```python
from build123d import *

# Parameters (mm, degrees)
F0_W         = 9.525
F0_H         = 50.8
F0_R         = 3.175
F0_W_2       = 31.75
F0_H_2       = 31.75
F0_R_2       = 6.35
F0_H_3       = 38.1
F1_DEPTH     = 12.7
F2_R         = 3.175
F3_W         = 9.525
F3_H         = 12.7
F1_FACE1_R   = 6.35
F1_FACE1_R_2 = 3.175
F4_DEPTH     = 1.5875
F5_DEPTH     = 1.5875
F6_DEPTH     = 1.5875


with BuildPart() as f1:
    # F0 (on Right) → F1 (new body)
    with BuildSketch(Plane.YZ):
        with Locations((134.9375, 25.4)):
            Rectangle(F0_W, F0_H)
        with BuildLine():
            Line((139.7, 50.8), (139.7, 0))
            Line((139.7, 0), (304.8, 0))
            Line((304.8, 0), (304.8, 19.05))
            Line((304.8, 19.05), (266.7, 19.05))
            Line((266.7, 19.05), (266.7, 40.9178125))
            Line((266.7, 40.9178125), (290.922752809, 52.7264044944))
            ThreePointArc((290.922752809, 52.7264044944), (299.6985955056, 78.197752809), (274.227247191, 86.9735955056))
            Line((274.227247191, 86.9735955056), (200.025, 50.8))
            Line((200.025, 50.8), (139.7, 50.8))
        make_face()
        with Locations((230.1875, 12.7)):
            Circle(F0_R, mode=Mode.SUBTRACT)
        with Locations((165.1, 25.4)):
            Rectangle(F0_W_2, F0_H_2, mode=Mode.SUBTRACT)
        with BuildLine():
            Line((190.5, 38.1), (200.025, 38.1))
            ThreePointArc((200.025, 38.1), (203.2, 34.925), (200.025, 31.75))
            Line((200.025, 31.75), (200.025, 19.05))
            ThreePointArc((200.025, 19.05), (203.2, 15.875), (200.025, 12.7))
            Line((200.025, 12.7), (190.5, 12.7))
            ThreePointArc((190.5, 12.7), (187.325, 15.875), (190.5, 19.05))
            Line((190.5, 19.05), (190.5, 31.75))
            ThreePointArc((190.5, 31.75), (187.325, 34.925), (190.5, 38.1))
        make_face(mode=Mode.SUBTRACT)
        with Locations((282.575, 69.85)):
            Circle(F0_R_2, mode=Mode.SUBTRACT)
        with BuildLine():
            Line((73.025, 38.1), (73.025, 0))
            Line((73.025, 0), (130.175, 0))
            Line((130.175, 0), (130.175, 50.8))
            Line((130.175, 50.8), (73.025, 50.8))
            Line((73.025, 50.8), (73.025, 44.6185247588))
            ThreePointArc((73.025, 44.6185247588), (76.2842623794, 41.3592623794), (73.025, 38.1))
        make_face()
        with Locations((104.775, 25.4)):
            Rectangle(F0_W_2, F0_H_2, mode=Mode.SUBTRACT)
        with Locations((68.2625, 19.05)):
            Rectangle(F0_W, F0_H_3)
        with BuildLine():
            Line((0, 41.275), (0, 0))
            Line((0, 0), (63.5, 0))
            Line((63.5, 0), (63.5, 38.1))
            ThreePointArc((63.5, 38.1), (60.325, 41.275), (63.5, 44.45))
            Line((63.5, 44.45), (63.5, 50.8))
            Line((63.5, 50.8), (50.8, 50.8))
            Line((50.8, 50.8), (50.8, 25.4))
            ThreePointArc((50.8, 25.4), (44.45, 19.05), (38.1, 25.4))
            Line((38.1, 25.4), (38.1, 50.8))
            Line((38.1, 50.8), (26.7157145118, 50.8))
            Line((26.7157145118, 50.8), (0, 41.275))
        make_face()
    extrude(amount=F1_DEPTH)

    # F2
    f2_edges = [f1.edges().sort_by_distance(p)[0] for p in [
        (6.35, 200.025, 50.8),
        (6.35, 266.7, 40.917813),
        (6.35, 266.7, 19.05),
        (6.35, 304.8, 19.05),
        (6.35, 304.8, 0),
        (6.35, 149.225, 41.275),
        (6.35, 88.9, 41.275),
        (6.35, 180.975, 9.525),
        (6.35, 180.975, 41.275),
        (6.35, 120.65, 41.275),
        (6.35, 149.225, 9.525),
        (6.35, 88.9, 9.525),
        (6.35, 120.65, 9.525),
        (6.35, 26.715715, 50.8),
    ]]
    fillet(f2_edges, radius=F2_R)

    # F3 (on face) + F1_face1 (on face) → F4 (cut)
    with BuildSketch(Plane(origin=(0, 0, 0), x_dir=(0, -1, 0), z_dir=(-1, 0, 0))):
        with Locations((-195.2625, 6.35)):
            Rectangle(F3_W, F3_H)
        with BuildLine():
            Line((-190.5, 38.1), (-190.5, 50.8))
            Line((-190.5, 50.8), (-199.2923076923, 50.8))
            ThreePointArc((-199.2923076923, 50.8), (-199.6611512097, 50.8214972713), (-200.025, 50.8856979781))
            Line((-200.025, 50.8856979781), (-200.025, 38.1))
            Line((-200.025, 38.1), (-190.5, 38.1))
        make_face()
    with BuildSketch(Plane(origin=(12.7, 165.3857306848, 30.2558551576), x_dir=(0, 1, 0), z_dir=(1, 0, 0))):
        with BuildLine():
            Line((139.4142693152, -27.0808551576), (139.4142693152, -14.3808551576))
            ThreePointArc((139.4142693152, -14.3808551576), (138.4843333455, -12.1357911273), (136.2392693152, -11.2058551576))
            Line((136.2392693152, -11.2058551576), (104.4892693152, -11.2058551576))
            ThreePointArc((104.4892693152, -11.2058551576), (102.2442052849, -10.2759191878), (101.3142693152, -8.0308551576))
            Line((101.3142693152, -8.0308551576), (101.3142693152, 8.6775823424))
            ThreePointArc((101.3142693152, 8.6775823424), (101.7968747, 10.3603289769), (103.0979771804, 11.5315149267))
            Line((103.0979771804, 11.5315149267), (125.5370221242, 22.4705493368))
            ThreePointArc((125.5370221242, 22.4705493368), (134.3128648208, 47.9418976514), (108.8415165062, 56.717740348))
            Line((108.8415165062, 56.717740348), (35.2978691423, 20.8652122582))
            ThreePointArc((35.2978691423, 20.8652122582), (34.6205059413, 20.6254527961), (33.9065770075, 20.5441448424))
            Line((33.9065770075, 20.5441448424), (-92.3607306848, 20.5441448424))
            Line((-92.3607306848, 20.5441448424), (-92.3607306848, 14.3626696012))
            ThreePointArc((-92.3607306848, 14.3626696012), (-89.1014683054, 11.1034072218), (-92.3607306848, 7.8441448424))
            Line((-92.3607306848, 7.8441448424), (-101.8857306848, 7.8441448424))
            ThreePointArc((-101.8857306848, 7.8441448424), (-105.0607306848, 11.0191448424), (-101.8857306848, 14.1941448424))
            Line((-101.8857306848, 14.1941448424), (-101.8857306848, 20.5441448424))
            Line((-101.8857306848, 20.5441448424), (-114.5857306848, 20.5441448424))
            Line((-114.5857306848, 20.5441448424), (-114.5857306848, -4.8558551576))
            ThreePointArc((-114.5857306848, -4.8558551576), (-120.9357306848, -11.2058551576), (-127.2857306848, -4.8558551576))
            Line((-127.2857306848, -4.8558551576), (-127.2857306848, 20.5441448424))
            Line((-127.2857306848, 20.5441448424), (-138.120948876, 20.5441448424))
            ThreePointArc((-138.120948876, 20.5441448424), (-138.661985551, 20.4977075022), (-139.1871958927, 20.3597538606))
            Line((-139.1871958927, 20.3597538606), (-165.3857306848, 11.0191448424))
            Line((-165.3857306848, 11.0191448424), (-165.3857306848, -30.2558551576))
            Line((-165.3857306848, -30.2558551576), (136.2392693152, -30.2558551576))
            ThreePointArc((136.2392693152, -30.2558551576), (138.4843333455, -29.3259191878), (139.4142693152, -27.0808551576))
        make_face()
        with Locations((117.1892693152, 39.5941448424)):
            Circle(F1_FACE1_R, mode=Mode.SUBTRACT)
        with Locations((64.8017693152, -17.5558551576)):
            Circle(F1_FACE1_R_2, mode=Mode.SUBTRACT)
        with BuildLine():
            Line((34.6392693152, -17.5558551576), (25.1142693152, -17.5558551576))
            ThreePointArc((25.1142693152, -17.5558551576), (21.9392693152, -14.3808551576), (25.1142693152, -11.2058551576))
            Line((25.1142693152, -11.2058551576), (25.1142693152, 1.4941448424))
            ThreePointArc((25.1142693152, 1.4941448424), (21.9392693152, 4.6691448424), (25.1142693152, 7.8441448424))
            Line((25.1142693152, 7.8441448424), (34.6392693152, 7.8441448424))
            ThreePointArc((34.6392693152, 7.8441448424), (37.8142693152, 4.6691448424), (34.6392693152, 1.4941448424))
            Line((34.6392693152, 1.4941448424), (34.6392693152, -11.2058551576))
            ThreePointArc((34.6392693152, -11.2058551576), (37.8142693152, -14.3808551576), (34.6392693152, -17.5558551576))
        make_face(mode=Mode.SUBTRACT)
        with BuildLine():
            Line((-16.1607306848, -17.5558551576), (-16.1607306848, 7.8441448424))
            ThreePointArc((-16.1607306848, 7.8441448424), (-15.2307947151, 10.0892088727), (-12.9857306848, 11.0191448424))
            Line((-12.9857306848, 11.0191448424), (12.4142693152, 11.0191448424))
            ThreePointArc((12.4142693152, 11.0191448424), (14.6593333455, 10.0892088727), (15.5892693152, 7.8441448424))
            Line((15.5892693152, 7.8441448424), (15.5892693152, -17.5558551576))
            ThreePointArc((15.5892693152, -17.5558551576), (14.6593333455, -19.8009191878), (12.4142693152, -20.7308551576))
            Line((12.4142693152, -20.7308551576), (-12.9857306848, -20.7308551576))
            ThreePointArc((-12.9857306848, -20.7308551576), (-15.2307947151, -19.8009191878), (-16.1607306848, -17.5558551576))
        make_face(mode=Mode.SUBTRACT)
        with BuildLine():
            Line((-47.9107306848, -20.7308551576), (-73.3107306848, -20.7308551576))
            ThreePointArc((-73.3107306848, -20.7308551576), (-75.5557947151, -19.8009191878), (-76.4857306848, -17.5558551576))
            Line((-76.4857306848, -17.5558551576), (-76.4857306848, 7.8441448424))
            ThreePointArc((-76.4857306848, 7.8441448424), (-75.5557947151, 10.0892088727), (-73.3107306848, 11.0191448424))
            Line((-73.3107306848, 11.0191448424), (-47.9107306848, 11.0191448424))
            ThreePointArc((-47.9107306848, 11.0191448424), (-45.6656666545, 10.0892088727), (-44.7357306848, 7.8441448424))
            Line((-44.7357306848, 7.8441448424), (-44.7357306848, -17.5558551576))
            ThreePointArc((-44.7357306848, -17.5558551576), (-45.6656666545, -19.8009191878), (-47.9107306848, -20.7308551576))
        make_face(mode=Mode.SUBTRACT)
    extrude(amount=-F4_DEPTH, dir=(-1, 0, 0), mode=Mode.SUBTRACT)

    # F0 (on Right) → F5 (cut)
    with BuildSketch(Plane.YZ):
        with Locations((134.9375, 25.4)):
            Rectangle(F0_W, F0_H)
    extrude(amount=F5_DEPTH, mode=Mode.SUBTRACT)

    # F0 (on Right) → F6 (cut)
    with BuildSketch(Plane.YZ):
        with Locations((68.2625, 19.05)):
            Rectangle(F0_W, F0_H_3)
    extrude(amount=F6_DEPTH, mode=Mode.SUBTRACT)


solid = f1.part
```
Here's how the part is built. I have some questions about the finished solid (model axes, mm). A direction names the side the tool comes from. Coordinates: 2 decimals unless noted, no trailing zeros. Order: outer loops, then holes, each group sorted by start corner. A loop starts at its lowest first (then second) coordinate and runs counter-clockwise, first axis right, second up.
1) We'd pull the mould along Z, two halves only. Please class faces 4 (the face through (6, 33, 50.8)), 5 (the face through (1.588, 68, 19)), 6 (the face through (6, 88.9, 25)): +Z half, -Z half, draft (parallel to the pull), parting line (faces both ways), or undercut.
2) Imagine slicing it at C-C on y = 249. List the corners of the cut face in (x, z) for me.
3) Imagine slicing it at A-A on z = 69.85. List the corners of the cut face in (x, y) for me (3 decimals), and give its area (3 significant figures).
4) Will these pins go through, and if not, where does the flat tip stop? pin 1 (7.5 mm diameter, centred on y = 282.575, z = 69.85, fed in from -X) (1 decimal); pin 2 (5 mm diameter, centred on x = 5.5, y = 196, fed in from +Z); pin 3 (4 mm diameter, centred on x = 9, y = 279.5, fed in from +Z); pin 4 (2 mm diameter, centred on x = 7, z = 78, fed in from +Y).
5) Which directions (+Z, -Z, +X, -X, +Y, -Y) give clear straight access to the entire face, cutting with the end or side of a thin tool? Please do faces 1 (the face through (6, 57, 50.8)), 2 (the face through (6, 165, 9.525)), 3 (the face through (1.588, 195, 45)).
6) I need wall thicknesses on line 1 (Y direction, x = 9.5, z = 30) (3 decimals); line 2 (Z direction, x = 9.25, y = 108) (3 decimals); line 3 (Z direction, x = 10, y = 194). Which ranges of each line are inside material? Lowest first, please.
7) Imagine slicing it at B-B on x = 5. State how many separate pieces and enclosed holes the cut face has, and give its area (3 significant figures).
8) Imagine slicing it at D-D on y = 18. List the corners of the cut face in (x, z) for me.
Response values:
1. face 4: +Z half
1. face 5: draft
1. face 6: undercut
2. outline: (0, 0) - (12.7, 0) - (12.7, 74.68) - (0, 74.68) - close
3. outline: (0, 239.102) - (12.7, 239.102) - (12.7, 276.225) - (0, 276.225) - close; (0, 288.925) - (12.7, 288.925) - (12.7, 301.625) - (0, 301.625) - close
3. area: 633 mm2
4. pin 1: passes through
4. pin 2: stops at z = 50.8
4. pin 3: stops at z = 88.87
4. pin 4: stops at y = 300.23
5. face 1: +Z, +X, -X, -Y
5. face 2: +X, -X
5. face 3: +Z, -Z, -X
6. line 1: y = 0 to 38.1, 50.8 to 88.9, 120.65 to 149.225, 180.975 to 190.5, 200.025 to 266.7
6. line 2: z = 0 to 9.525, 41.275 to 50.8
6. line 3: z = 0 to 12.7, 38.1 to 50.8
7. separate pieces: 1
7. enclosed holes: 5
7. area: 13,500 mm2
8. outline: (0, 0) - (12.7, 0) - (12.7, 47.69) - (0, 47.69) - close
